Read the model definition and answer for the solid it produces. Units are mm, in the model's axes. Round coordinates to 2 decimals unless told otherwise and drop trailing zeros. Order: outer loops, then holes, each group sorted by start corner. A loop starts at its lowest first (then second) coordinate and runs counter-clockwise, first axis right, second up. Notation, with made-up numbers: (0.25, 32) - (53.25, 32) arc R27 cw to (53.25, 51) - close; hole circle Ø5 at (-26.5, -7). An arc over 180 degrees is marked (long way). Put each result on its own line as item: value. Start each with the question number.
Q1. Section A-A on x = 0 is taken. Give the vertices of the cut face in (y, z).
Q2. For a pull along Z with two mould halves and no side action, classify faces 1 (the face through (-2, 6, -2.5)), 2 (the face through (-2, 6, 2.5)), 3 (the face through (4.77, -8.22, -0.04)) as pulls with the +Z half, pulls with the -Z half, needs draft (parallel to the pull), parting line crosses it, or undercut.
Q3. Find the intervals of material crossed by line 1 along Y through (x, z) = (0, 0.7); line 2 along Y through (x, z) = (5.5, 0); line 3 along X through (y, z) = (-0.25, -1), in increasing order. Write a range as from..to.
Q4. Section B-B on z = 1.75 is taken. Give the vertices of the cut face in (x, y).
Q5. This flat-tipped pin is pushed along its axis until it touches: pin 1 Ø1.5 at (y, z) = (-5, -2) entering from +X. Where does it stop, or does it pass through?
Q6. Section D-D on x = -6.25 is taken. Give the vertices of the cut face in (y, z), then the cut area to 3 significant figures.
Q7. Section C-C on y = 0 is taken. Give the vertices of the cut face in (x, z).
Autodesk Inventor part; units mm, degrees
ref_plane "YZ Plane" through (0, 0, 0) normal (1, 0, 0) x (0, 1, 0)
ref_plane "XZ Plane" through (0, 0, 0) normal (0, 1, 0) x (-1, 0, 0)
ref_plane "XY Plane" through (0, 0, 0) normal (0, 0, 1) x (1, 0, 0)
sketch "Sketch1" plane through (0, 0, 0) normal (0, 0, 1) x (1, 0, 0)
  line L0 (9.815, 0) -> (4.9075, -8.5)
  line L1 (4.9075, -8.5) -> (-4.9075, -8.5)
  line L2 (-4.9075, -8.5) -> (-9.815, 0)
  line L3 (-9.815, 0) -> (-4.9075, 8.5)
  line L4 (-4.9075, 8.5) -> (4.9075, 8.5)
  line L5 (4.9075, 8.5) -> (9.815, 0)
  point P0 (0, 0)
  point P1 (0, 0)
  dimension "d0" = 17
extrude "Extrusion1" add sketch "Sketch1" along normal mid plane 5
sketch "Sketch2" plane through (0, 0, 2.5) normal (0, 0, 1) x (1, 0, 0)
  circle A0 centre (0, 0) radius 6
  dimension "d3" = 12
extrude "Extrusion2" cut sketch "Sketch2" against normal through all
fillet "Fillet1" radius 2 6 edges at (4.9075, -8.5, 0) (-4.9075, -8.5, 0) (-9.815, 0, 0) (-4.9075, 8.5, 0) (4.9075, 8.5, 0) (9.815, 0, 0)
properties part number "M12_NUT_1.262.1200.50"
Findings:
1. outline: (-8.5, -2.5) - (-6, -2.5) - (-6, 2.5) - (-8.5, 2.5) - close; (6, -2.5) - (8.5, -2.5) - (8.5, 2.5) - (6, 2.5) - close
2. face 1: pulls with the -Z half
2. face 2: pulls with the +Z half
2. face 3: needs draft
3. line 1: -8.5..-6, 6..8.5
3. line 2: -7.47..-2.4, 2.4..7.47
3. line 3: -9.49..-5.99, 5.99..9.49
4. outline: (-9.24, -1) - (-5.48, -7.5) arc R2 ccw to (-3.75, -8.5) - (3.75, -8.5) arc R2 ccw to (5.48, -7.5) - (9.24, -1) arc R2 ccw to (9.24, 1) - (5.48, 7.5) arc R2 ccw to (3.75, 8.5) - (-3.75, 8.5) arc R2 ccw to (-5.48, 7.5) - (-9.24, 1) arc R2 ccw to start; hole circle Ø12 at (0, 0)
5. pin 1: x = 7.36
6. outline: (-6.17, -2.5) - (6.17, -2.5) - (6.17, 2.5) - (-6.17, 2.5) - close
6. area: 61.7 mm2
7. outline: (-9.51, -2.5) - (-6, -2.5) - (-6, 2.5) - (-9.51, 2.5) - close; (6, -2.5) - (9.51, -2.5) - (9.51, 2.5) - (6, 2.5) - close
